```python
from build123d import *

# Parameters (mm, degrees)
SKETCH1_R           = 6
SKETCH1_R_2         = 1.5
BOSS_EXTRUDE1_DEPTH = 4


with BuildPart() as part:
    # Sketch1 → Boss-Extrude1 (new body)
    with BuildSketch(Plane(origin=(0, 0, 0), x_dir=(1, 0, 0), z_dir=(0, 1, 0))):
        Circle(SKETCH1_R)
        Circle(SKETCH1_R_2, mode=Mode.SUBTRACT)
    extrude(amount=BOSS_EXTRUDE1_DEPTH)

    # Sketch6 → Cut-Revolve1 (revolve, cut)
    with BuildSketch(Plane.XY):
        Polygon((6, 0.5), (6, 3.5), (4.8, 2.5), (4.8, 1.5), align=None)
    revolve(axis=Axis((0, 4, 0), (0, -1, 0)), mode=Mode.SUBTRACT)


solid = part.part
```
The model under review builds one solid part; all positions refer to its coordinate system, in mm. A direction names the side the tool comes from. Coordinates: 2 decimals unless noted, no trailing zeros. Order: outer loops, then holes, each group sorted by start corner. A loop starts at its lowest first (then second) coordinate and runs counter-clockwise, first axis right, second up. Notation, with made-up numbers: (13.5, 49.5) -> (47.5, 49.5) arc R28 cw to (47.5, 72.5) -> close; hole circle Ø7 at (-24, -19.5). An arc over 180 degrees is marked (long way). Answer in a Markdown table with one row per item. Add a question column.
Item 1: Mouldability with a two-part tool opening along X and no side actions: class faces 1 (the conical face through (-3.9, 1.4, -3)), 2 (the flat face through (1.2, 4, 1.2)), 3 (the cylindrical face through (-1.5, 1.97, -0.07)) as +X half, -X half, draft (parallel to the pull), parting line (faces both ways), or undercut.
Item 2: Clearance check with flat-ended pins moving along their axes: pin 1 (1.5 mm diameter, centred on y = 1, z = -4.5, fed in from +X); pin 2 (1.5 mm diameter, centred on x = -1.5, y = 1.5, fed in from +Z). State where each tip first meets the part, or that it passes through.
Item 3: We need section B-B on z = 0. Write out the cut boundary in (x, y).
Item 4: To check wall thickness, follow probe 1 along Z at (x, y) = (0, 1.7); probe 2 along Y at (x, z) = (-2.25, 5.25); probe 3 along Z at (x, y) = (0, 3). State the ranges of each line that lie inside material, in increasing order.
Item 5: We need section C-C on y = 3.75. Write out the cut boundary in (x, z).
Item 6: We need section D-D on y = 2.3. Write out the cut boundary in (x, z).
Item 7: Machinability: for faces 4 (the cylindrical face through (2.58, 1.99, 4.05)), 5 (the cylindrical face through (-5.994, 3.746, -0.264)), which of the approach directions +Z, -Z, +X, -X, +Y, -Y give a long, thin tool a straight path to every point of the face, cutting with its end or side? Answer none if there is none.
Item 8: We need section A-A on x = 0. Write out the cut boundary in (y, z).
Final values:
| question | item | result |
|---|---|---|
| 1 | face 1 | parting line |
| 1 | face 2 | draft |
| 1 | face 3 | undercut |
| 2 | pin 1 | stops at x = 4.52 |
| 2 | pin 2 | stops at z = 5.52 |
| 3 | outline | (-6, 0) -> (-1.5, 0) -> (-1.5, 4) -> (-6, 4) -> (-6, 3.5) -> (-4.8, 2.5) -> (-4.8, 1.5) -> (-6, 0.5) -> close; (1.5, 0) -> (6, 0) -> (6, 0.5) -> (4.8, 1.5) -> (4.8, 2.5) -> (6, 3.5) -> (6, 4) -> (1.5, 4) -> close |
| 4 | probe 1 | z = -4.8 to -1.5, 1.5 to 4.8 |
| 4 | probe 2 | y = 0 to 0.74, 3.26 to 4 |
| 4 | probe 3 | z = -5.4 to -1.5, 1.5 to 5.4 |
| 5 | outline | circle Ø12 at (0, 0); hole circle Ø3 at (0, 0) |
| 6 | outline | circle Ø9.6 at (0, 0); hole circle Ø3 at (0, 0) |
| 7 | face 4 | none |
| 7 | face 5 | +Y, -Y |
| 8 | outline | (0, -6) -> (0.5, -6) -> (1.5, -4.8) -> (2.5, -4.8) -> (3.5, -6) -> (4, -6) -> (4, -1.5) -> (0, -1.5) -> close; (0, 1.5) -> (4, 1.5) -> (4, 6) -> (3.5, 6) -> (2.5, 4.8) -> (1.5, 4.8) -> (0.5, 6) -> (0, 6) -> close |
